Design review of the part built by this model. Coordinates are the model's own, in mm. A direction names the side the tool comes from. Round coordinates to 2 decimals unless told otherwise and drop trailing zeros. Loops run counter-clockwise (first coordinate to the right, second up) from the corner with the lowest first, then second, coordinate; pieces in that order, holes last. Notation, with made-up numbers: (7.25, 34) - (27.25, 34) arc R23 cw to (27.25, 73) - close; hole circle Ø4 at (-22, 52.25). An arc over 180 degrees is marked (long way). Return JSON: item names as keys, results as strings. Group by question number.
from build123d import *

# Parameters (mm, degrees)
SKETCH_1_R          = 4.925
EXTRUDE_1_DEPTH     = 6.08
SKETCH_2_R          = 3.875
CUT_EXTRUDE_1_DEPTH = 5.08
FILLET_1_R          = 0.5
CUT_EXTRUDE_2_DEPTH = 2


with BuildPart() as part:
    # Эскиз1 → Бобышка-Вытянуть1 (new body)
    with BuildSketch(Plane(origin=(0, 0, 0), x_dir=(1, 0, 0), z_dir=(0, 1, 0))):
        Circle(SKETCH_1_R)
    extrude(amount=EXTRUDE_1_DEPTH)

    # Эскиз2 → Вырез-Вытянуть1 (cut)
    with BuildSketch(Plane(origin=(0, 6.08, 0), x_dir=(1, 0, 0), z_dir=(0, 1, 0))):
        Circle(SKETCH_2_R)
    extrude(amount=-CUT_EXTRUDE_1_DEPTH, mode=Mode.SUBTRACT)

    # Скругление1
    fillet_1_edges = [part.edges().sort_by_distance(p)[0] for p in [
        (-4.925, 6.08, 0),
    ]]
    fillet(fillet_1_edges, radius=FILLET_1_R)

    # Эскиз3 → Вырез-Вытянуть2 (cut, through all)
    with BuildSketch(Plane(origin=(0, 1, 0), x_dir=(1, 0, 0), z_dir=(0, 1, 0))):
        with BuildLine():
            Line((2.875, 0.5), (0.5, 0.5))
            Line((0.5, 0.5), (0.5, 2.875))
            ThreePointArc((0.5, 2.875), (0, 3.375), (-0.5, 2.875))
            Line((-0.5, 2.875), (-0.5, 0.5))
            Line((-0.5, 0.5), (-2.875, 0.5))
            ThreePointArc((-2.875, 0.5), (-3.375, 0), (-2.875, -0.5))
            Line((-2.875, -0.5), (-0.5, -0.5))
            Line((-0.5, -0.5), (-0.5, -2.875))
            ThreePointArc((-0.5, -2.875), (0, -3.375), (0.5, -2.875))
            Line((0.5, -2.875), (0.5, -0.5))
            Line((0.5, -0.5), (2.875, -0.5))
            ThreePointArc((2.875, -0.5), (3.375, 0), (2.875, 0.5))
        make_face()
    extrude(amount=-CUT_EXTRUDE_2_DEPTH, mode=Mode.SUBTRACT)


solid = part.part
Q1. Insertion check: pin 1 Ø1.1 at (y, z) = (0.5, 1.5) entering from -X; pin 2 Ø0.5 at (x, y) = (2, 0.5) entering from -Z; pin 3 Ø0.8 at (y, z) = (0.5, 1.5) entering from +X; pin 4 Ø1.5 at (y, z) = (2.5, 0.5) entering from -X (3 decimals). Each pin has a flat end and moves straight along its axis. Give the tip position at first contact, or say it passes through.
Q2. Add section C-C, the plane y = 4. State the section outline as (x, z) points (3 decimals), plus the area to 3 significant figures.
Q3. Add section A-A, the plane z = 0. State the section outline as (x, y) points (3 decimals), plus the area to 3 significant figures.
Q4. Draft analysis for pull direction X (two halves, no side actions). For faces 4 (the cylindrical face through (-3.908, 2.751, 2.997)), 5 (the flat face through (3, 6.08, 3)), 6 (the cylindrical face through (3.375, 0.507, 0.011)), state which applies: pulls with the +X half, pulls with the -X half, needs draft (parallel to the pull), parting line crosses it, or undercut.
Q5. For line 1 (X direction, y = 5.25, z = 0) (3 decimals); line 2 (Z direction, x = 2.75, y = 2.5), list the stretches that pass through material, from the lowest coordinate up.
Q6. Tool access review of faces 1 (the flat face through (1, 0, 1)), 2 (the cylindrical face through (-0.504, 3.576, -3.842)), 3 (the flat face through (-1.7, 0.5, -0.5)): name each direction out of +Z, -Z, +X, -X, +Y, -Y from which nothing blocks a thin tool from reaching the whole face with its end or side.
Q7. Add section B-B, the plane x = 0. State the section outline as (y, z) points (3 decimals), plus the area to 3 significant figures.
Evaluation:
{
 "1": {"pin 1": "x = -4.83", "pin 2": "z = -4.6", "pin 3": "x = 4.8", "pin 4": "x = -4.925"},
 "2": {"outline": "circle Ø9.85 at (0, 0); hole circle Ø7.75 at (0, 0)", "area": "29.0 mm²"},
 "3": {"outline": "(-4.925, 0) - (-3.375, 0) - (-3.375, 1) - (-3.875, 1) - (-3.875, 6.08) - (-4.425, 6.08) arc R0.5 ccw to (-4.925, 5.58) - close; (3.375, 0) - (4.925, 0) - (4.925, 5.58) arc R0.5 ccw to (4.425, 6.08) - (3.875, 6.08) - (3.875, 1) - (3.375, 1) - close", "area": "13.7 mm²"},
 "4": {"face 4": "parting line crosses it", "face 5": "needs draft", "face 6": "undercut"},
 "5": {"line 1": "-4.925 to -3.875, 3.875 to 4.925", "line 2": "-4.09 to -2.73, 2.73 to 4.09"},
 "6": {"face 1": "+Z, -Z, +X, -X, -Y", "face 2": "+Y", "face 3": "+Y, -Y"},
 "7": {"outline": "(0, -4.925) - (5.58, -4.925) arc R0.5 ccw to (6.08, -4.425) - (6.08, -3.875) - (1, -3.875) - (1, -3.375) - (0, -3.375) - close; (0, 3.375) - (1, 3.375) - (1, 3.875) - (6.08, 3.875) - (6.08, 4.425) arc R0.5 ccw to (5.58, 4.925) - (0, 4.925) - close", "area": "13.7 mm²"}
}
